CAD build for the part. Positions are in the model's coordinates, mm. Face numbers are marked on the shaded views. A direction names the side the tool comes from. Give positions to 0.01 mm unless a question says otherwise; leave off trailing zeros. Loops run counter-clockwise (first coordinate to the right, second up) from the corner with the lowest first, then second, coordinate; pieces in that order, holes last. Notation, with made-up numbers: M 65,-9 L 103,-9 A25 ccw 103,19 Z; hole C -38.5,41.25 d7. An arc over 180 degrees is marked long. Answer as CSV lines item,"result".
```python
from build123d import *

# Parameters (mm, degrees)
F1_DEPTH  = 2.5
F3_DEPTH  = 2.7
F4_R      = 1
F5_R      = 5
F6_W      = 4
F6_H      = 2
F6_H_2    = 4
F7_DEPTH  = 2
F8_R      = 1.25
F9_DEPTH  = 6
F10_R     = 2.25
F11_DEPTH = 2.5


with BuildPart() as f1:
    # F0 (on Top) → F1 (new body)
    with BuildSketch(Plane.XY):
        Polygon((55, 0), (4, 0), (0, -10), (0, -47), (59, -47), (59, -10), align=None)
    extrude(amount=F1_DEPTH)

    # F2 (on face) → F3 (join)
    with BuildSketch(Plane.XY.offset(2.5)):
        with BuildLine():
            Line((0, -39.5), (0, -47))
            Line((0, -47), (59, -47))
            Line((59, -47), (59, -39.5))
            Line((59, -39.5), (53.5, -32))
            Line((53.5, -32), (53.5, -4))
            ThreePointArc((53.5, -4), (52.3284271247, -1.1715728753), (49.5, 0))
            Line((49.5, 0), (9.5, 0))
            ThreePointArc((9.5, 0), (6.6715728753, -1.1715728753), (5.5, -4))
            Line((5.5, -4), (5.5, -32))
            Line((5.5, -32), (0, -39.5))
        make_face()
    extrude(amount=F3_DEPTH)

    # F4
    f4_edges = [f1.edges().sort_by_distance(p)[0] for p in [
        (0, -47, 2.6),
        (59, -47, 2.6),
        (4, 0, 1.25),
        (55, 0, 1.25),
        (59, -10, 1.25),
        (0, -10, 1.25),
    ]]
    fillet(f4_edges, radius=F4_R)

    # F5
    f5_edges = [f1.edges().sort_by_distance(p)[0] for p in [
        (0, -39.5, 3.85),
        (59, -39.5, 3.85),
        (53.5, -32, 3.85),
        (5.5, -32, 3.85),
    ]]
    fillet(f5_edges, radius=F5_R)

    # F6 (on face) → F7 (join)
    with BuildSketch(Plane.XY.offset(5.2)):
        with Locations((11.5, -5)):
            Rectangle(F6_W, F6_H)
        with Locations((11.5, -41)):
            Rectangle(F6_W, F6_H_2)
        with Locations((47.5, -5)):
            Rectangle(F6_W, F6_H)
        with Locations((47.5, -41)):
            Rectangle(F6_W, F6_H_2)
    extrude(amount=F7_DEPTH)

    # F8 (on face) → F9 (cut)
    with BuildSketch(Plane.XY.offset(5.2)):
        with Locations((23.5, -13.5)):
            Circle(F8_R)
        with Locations((35.5, -13.5)):
            Circle(F8_R)
    extrude(amount=-F9_DEPTH, mode=Mode.SUBTRACT)

    # F10 (on face) → F11 (cut)
    with BuildSketch(Plane.XY):
        with Locations((35.5, -13.5)):
            Circle(F10_R)
        with Locations((23.5, -13.5)):
            Circle(F10_R)
    extrude(amount=F11_DEPTH, mode=Mode.SUBTRACT)


solid = f1.part
```
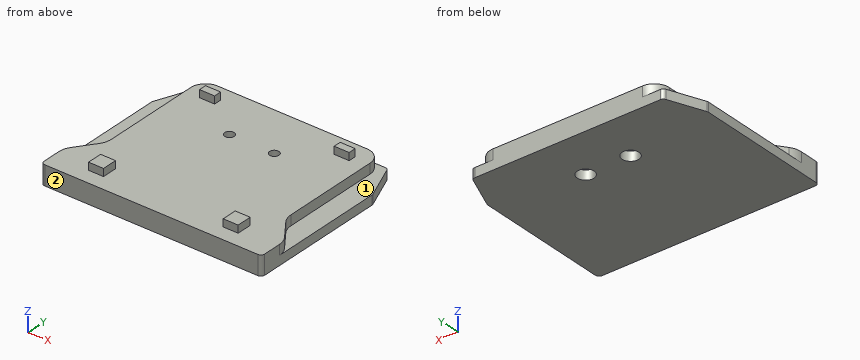
Q1. Cut at C-C (z = 6). Write the cut outline in (x, y).
Solution:
outline,"M 9.5,-43 L 13.5,-43 L 13.5,-39 L 9.5,-39 Z; M 9.5,-6 L 13.5,-6 L 13.5,-4 L 9.5,-4 Z; M 45.5,-43 L 49.5,-43 L 49.5,-39 L 45.5,-39 Z; M 45.5,-6 L 49.5,-6 L 49.5,-4 L 45.5,-4 Z"
Q2. Which spindle directions (+Z, -Z, +X, -X, +Y, -Y) get a long thin tool onto all of the face, cutting with end or side? Do the marked faces 1 and 2. Say none if no direction does.
Solution:
face 1,"+Z, +X, +Y"
face 2,"+Z, -Z, +X, -X, -Y"
Q3. Pin check, flat tips, straight feed: P1, Ø1, axis at x = 46.5, z = 6.5, coming from the +Y side; P2, Ø1.3, axis at x = 24.5, y = -14.5, coming from the -Z side; P3, Ø2, axis at x = 46.5, z = 6.5, coming from the -Y side. Stop position of each tip, or through.
Solution:
P1,"stops at y = -4"
P2,"stops at z = 2.5"
P3,"stops at y = -43"
Q4. Wall check: line 1 (Y direction, x = 23.5, z = 4.75); line 2 (X direction, y = -14.5, z = 0.75); line 3 (Y direction, x = 35.5, z = 1.9). Give the ranges that are in metal, low to high. Write a range as [from, to].
Solution:
line 1,"y = [-47, -14.75], [-12.25, 0]"
line 2,"x = [0, 21.48], [25.52, 33.48], [37.52, 59]"
line 3,"y = [-47, -15.75], [-11.25, 0]"
Q5. Cut at D-D (y = -23). Write the cut outline in (x, z), and give its area (3 significant figures).
Solution:
outline,"M 0,0 L 59,0 L 59,2.5 L 53.5,2.5 L 53.5,5.2 L 5.5,5.2 L 5.5,2.5 L 0,2.5 Z"
area,"277 mm²"
Q6. Cut at A-A (x = 35.5). Write the cut outline in (y, z).
Solution:
outline,"M -47,0 L -15.75,0 L -15.75,2.5 L -14.75,2.5 L -14.75,5.2 L -47,5.2 Z; M -12.25,2.5 L -11.25,2.5 L -11.25,0 L 0,0 L 0,5.2 L -12.25,5.2 Z"
Q7. Cut at B-B (y = -13.5). Write the cut outline in (x, z), and give its area (3 significant figures).
Solution:
outline,"M 0,0 L 21.25,0 L 21.25,2.5 L 22.25,2.5 L 22.25,5.2 L 5.5,5.2 L 5.5,2.5 L 0,2.5 Z; M 24.75,2.5 L 25.75,2.5 L 25.75,0 L 33.25,0 L 33.25,2.5 L 34.25,2.5 L 34.25,5.2 L 24.75,5.2 Z; M 36.75,2.5 L 37.75,2.5 L 37.75,0 L 59,0 L 59,2.5 L 53.5,2.5 L 53.5,5.2 L 36.75,5.2 Z"
area,"241 mm²"
